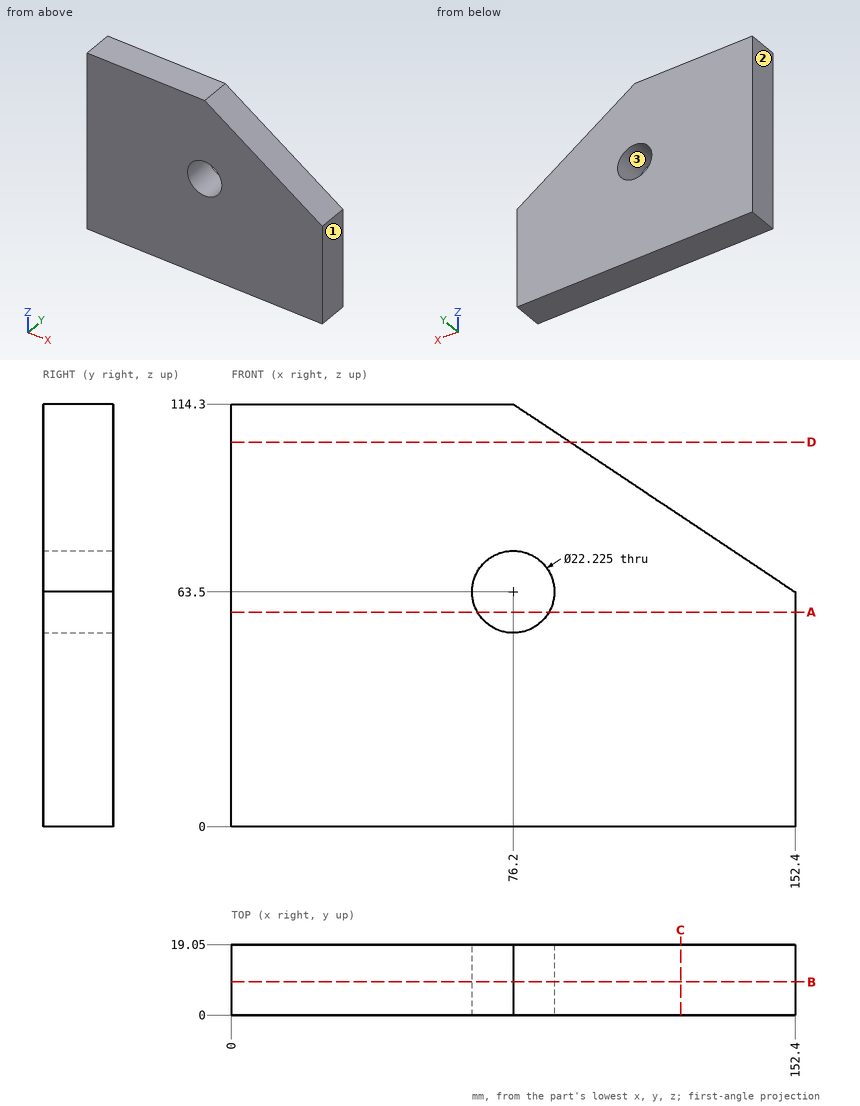
Geometry check sheet. Reference: drawing and pictorial views, mm from the part's lowest x, y, z. Give positions to 0.01 mm unless a question says otherwise; leave off trailing zeros. Order: outer loops, then holes, each group sorted by start corner. A loop starts at its lowest first (then second) coordinate and runs counter-clockwise, first axis right, second up. Notation, with made-up numbers: M 75.5,23.5 L 104.5,23.5 A22 cw 104.5,36.5 Z; hole C 43,45 d10. An arc over 180 degrees is marked long. Answer as CSV lines item,"result". Start each with the question number.
Item 1: Thickness scan on line 1 (Z direction, x = 76.2, y = 4.25); line 2 (X direction, y = 8.5, z = 63.5); line 3 (Z direction, x = 85.5, y = 17.5). Record the ranges inside material, lowest first. Write a range as [from, to].
Item 2: Cross-section at A-A on z = 58. Enter the section's corners in (x, y), plus the area to 3 significant figures.
Item 3: Cross-section at C-C on x = 121.5. Enter the section's corners in (y, z), plus the area to 3 significant figures.
Item 4: Cross-section at B-B on y = 9. Enter the section's corners in (x, z) (1 decimal), plus the area to 3 significant figures.
Item 5: Cross-section at D-D on z = 104. Enter the section's corners in (x, y).
Item 6: Gauge pin test, flat ends, axial feed: P1, Ø2, axis at y = 5, z = 80, coming from the +X side; P2, Ø6, axis at x = 95.5, y = 8.5, coming from the +Z side; P3, Ø3, axis at x = 83, y = 4.5, coming from the +Z side. Record the tip position at first contact, or that the pin passes through.
Item 7: Mould release check, pull along X, two halves, no side actions. Record for the marked faces 1, 2 and 3: +X half, -X half, draft (parallel to the pull), parting line (faces both ways), or undercut.
Established:
1,line 1,"z = [0, 52.39], [74.61, 114.3]"
1,line 2,"x = [0, 65.09], [87.31, 152.4]"
1,line 3,"z = [0, 57.42], [69.58, 108.1]"
2,outline,"M 0,0 L 66.54,0 L 66.54,19.05 L 0,19.05 Z; M 85.86,0 L 152.4,0 L 152.4,19.05 L 85.86,19.05 Z"
2,area,"2,540 mm^2"
3,outline,"M 0,0 L 19.05,0 L 19.05,84.1 L 0,84.1 Z"
3,area,"1,600 mm^2"
4,outline,"M 0,0 L 152.4,0 L 152.4,63.5 L 76.2,114.3 L 0,114.3 Z; hole C 76.2,63.5 d22.2"
4,area,"15,100 mm^2"
5,outline,"M 0,0 L 91.65,0 L 91.65,19.05 L 0,19.05 Z"
6,P1,"stops at x = 129.15"
6,P2,"stops at z = 103.43"
6,P3,"stops at z = 110.77"
7,face 1,"+X half"
7,face 2,"-X half"
7,face 3,"undercut"
